```python
from build123d import *

# Parameters (mm, degrees)
F1_DEPTH = 6
F2_R     = 10
F3_W     = 30.655736
F3_H     = 11
F4_DEPTH = 6
F5_R     = 1.525335
F6_DEPTH = 11.4


with BuildPart() as f1:
    # F0 (on Top) → F1 (new body)
    with BuildSketch(Plane.XY):
        Polygon((119.344264, 17.5), (-150, 17.5), (-150, -17.5), (119.344264, -17.5), (119.344264, -8.5), (0, -8.5), (0, -6.5), (150, -6.5), (150, 4.5), (0, 4.5), (0, 6.5), (119.344264, 6.5), align=None)
    extrude(amount=F1_DEPTH)

    # F2
    f2_edges = [f1.edges().sort_by_distance(p)[0] for p in [
        (-150, -17.5, 3),
        (-150, 17.5, 3),
    ]]
    fillet(f2_edges, radius=F2_R)

    # F3 (on face) → F4 (join)
    with BuildSketch(Plane.XY.offset(6)):
        with Locations((134.672132, -1)):
            Rectangle(F3_W, F3_H)
    extrude(amount=F4_DEPTH)

    # F5 (on face) → F6 (cut)
    with BuildSketch(Plane.XZ.offset(6.5)):
        with Locations((140.18032, 5.98348)):
            Circle(F5_R)
    extrude(amount=-F6_DEPTH, mode=Mode.SUBTRACT)


solid = f1.part
```
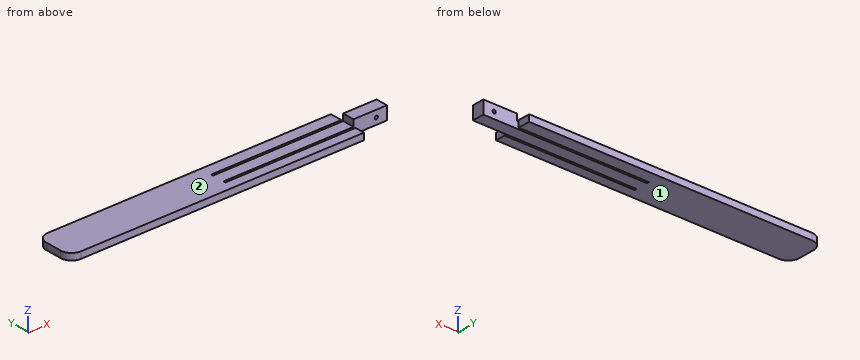
Geometry: final body of the model. Coordinates: model frame, mm. Face numbers are marked on the shaded views. A direction names the side the tool comes from. Coordinates: 2 decimals unless noted, no trailing zeros. Order: outer loops, then holes, each group sorted by start corner. A loop starts at its lowest first (then second) coordinate and runs counter-clockwise, first axis right, second up. Notation, with made-up numbers: (-29.5, 29.25) - (13.5, 29.25) arc R17 ccw to (13.5, 35.25) - close; hole circle Ø3 at (48, 1). An arc over 180 degrees is marked (long way). Return JSON: item names as keys, results as strings. Group by question number.
1. Cut plane D-D (y = -15). Output: boundary loops of the cut face in (x, z), plus the area to 3 significant figures.
2. Set-up query: the marked faces 1 and 2. Return all of +Z, -Z, +X, -X, +Y, -Y with unobstructed straight access to the full face (end or side cutting, diameter ignored); none if empty.
3. Cut plane B-B (y = -2). Output: boundary loops of the cut face in (x, z).
4. Material intervals for line 1 along Y through (x, z) = (40, 3); line 2 along Z through (x, y) = (99, 14.5); line 3 along X through (y, z) = (7, 3.5), sorted ascending. Write a range as [from, to].
5. Cut plane C-C (x = 122). Output: boundary loops of the cut face in (y, z), plus the area to 3 significant figures.
6. Pin query (flat end, axial travel): pin 1 (10 mm diameter, centred on x = 3.5, y = 6.5, fed in from +Z); pin 2 (2.5 mm diameter, centred on x = 140.18, z = 5.98, fed in from -Y); pin 3 (1.8 mm diameter, centred on y = 14, z = 3.5, fed in from +X); pin 4 (0.6 mm diameter, centred on y = -8, z = 4.5, fed in from +X). Return the tip coordinate at first contact, or that it passes through.
7. Cut plane A-A (x = 36). Output: boundary loops of the cut face in (y, z), plus the area to 3 significant figures.
Resolved:
{
 "1": {"outline": "(-146.61, 0) - (119.34, 0) - (119.34, 6) - (-146.61, 6) - close", "area": "1,600 mm²"},
 "2": {"face 1": "-Z, +X, -X, +Y, -Y", "face 2": "+Z, -X, +Y, -Y"},
 "3": {"outline": "(-150, 0) - (150, 0) - (150, 12) - (119.34, 12) - (119.34, 6) - (-150, 6) - close; hole circle Ø3.05 at (140.18, 5.98)"},
 "4": {"line 1": "y = [-17.5, -8.5], [-6.5, 4.5], [6.5, 17.5]", "line 2": "z = [0, 6]", "line 3": "x = [-150, 119.34]"},
 "5": {"outline": "(-6.5, 0) - (4.5, 0) - (4.5, 12) - (-6.5, 12) - close", "area": "132 mm²"},
 "6": {"pin 1": "stops at z = 6", "pin 2": "passes through", "pin 3": "stops at x = 119.34", "pin 4": "stops at x = 0"},
 "7": {"outline": "(-17.5, 0) - (-8.5, 0) - (-8.5, 6) - (-17.5, 6) - close; (-6.5, 0) - (4.5, 0) - (4.5, 6) - (-6.5, 6) - close; (6.5, 0) - (17.5, 0) - (17.5, 6) - (6.5, 6) - close", "area": "186 mm²"}
}
